The model under review builds one solid part; all positions refer to its coordinate system, in mm. A direction names the side the tool comes from. Round coordinates to 2 decimals unless told otherwise and drop trailing zeros. Loops run counter-clockwise (first coordinate to the right, second up) from the corner with the lowest first, then second, coordinate; pieces in that order, holes last. Notation, with made-up numbers: M 41.25,23 L 82.25,23 A26 cw 82.25,46 Z; hole C -10.5,61 d2. An arc over 180 degrees is marked long. Return JSON: item names as keys, results as strings. Group by question number.
Q1. Consider section B-B (y = -533.5). State the section outline as (x, z) points, and give its area (3 significant figures).
Q2. Consider section D-D (z = 609.5). State the section outline as (x, y) points, and give its area (3 significant figures).
Q3. Consider section A-A (x = 43). State the section outline as (y, z) points, and give its area (3 significant figures).
Q4. For faces 5 (the face through (-76.2, -9, 347)), 6 (the face through (-1, 590.55, 347)), list the 3-axis set-ups (+Z, -Z, +X, -X, +Y, -Y) from which the entire face can be reached by the end or side of a thin tool; tool diameter is ignored.
Q5. To check wall thickness, follow line 1 along Z through (x, y) = (61.5, 0); line 2 along X through (y, z) = (128.5, 73.5); line 3 along Y through (x, z) = (-68.75, 406.4). State the ranges of each line that lie inside material, in increasing order.
Q6. Consider section C-C (z = 268). State the section outline as (x, y) points.
Q7. Draft analysis for pull direction Y (two halves, no side actions). For faces 1 (the face through (62, 3, 0)), 2 (the face through (-1, -590.55, 347)), 3 (the face through (-1, 609.6, 347)), 4 (the face through (57.15, -8, 426)), state which applies: pulls with the +Y half, pulls with the -Y half, needs draft (parallel to the pull), parting line crosses it, or undercut.
from build123d import *

# Parameters (mm, degrees)
F0_W     = 152.4
F0_H     = 1219.2
F0_W_2   = 114.3
F0_H_2   = 1181.1
F1_DEPTH = 704.85
F3_DEPTH = 25.4
F5_DEPTH = 25.4


# Not quite as in the source:
# - a feature names something its author has since deleted; it is built from what else it names


with BuildPart() as f1:
    # F0 (on Top) → F1 (new body)
    with BuildSketch(Plane.XY):
        Rectangle(F0_W, F0_H)
        Rectangle(F0_W_2, F0_H_2, mode=Mode.SUBTRACT)
    extrude(amount=F1_DEPTH)

    # F2 (on face) → F3 (cut)
    with BuildSketch(Plane.YZ.offset(76.2)):
        with BuildLine():
            ThreePointArc((30.226, 596.9), (-21.3730095681, 618.2730095681), (0, 566.674))
            ThreePointArc((0, 566.674), (21.3730095681, 575.5269904319), (30.226, 596.9))
        make_face()
        Polygon((-133.35, 101.6), (0, 101.6), (133.35, 101.6), (133.35, 419.1), (0, 419.1), (-133.35, 419.1), align=None)
    extrude(amount=-F3_DEPTH, mode=Mode.SUBTRACT)

    # F4 (on face) → F5 (cut)
    with BuildSketch(Plane(origin=(-76.2, 0, 0), x_dir=(0, -1, 0), z_dir=(-1, 0, 0))):
        with BuildLine():
            ThreePointArc((30.226, 406.4), (-21.3730095681, 427.7730095681), (0, 376.174))
            ThreePointArc((0, 376.174), (21.3730095681, 385.0269904319), (30.226, 406.4))
        make_face()
    extrude(amount=-F5_DEPTH, mode=Mode.SUBTRACT)


solid = f1.part
Values:
{
 "1": {"outline": "M -76.2,0 L -57.15,0 L -57.15,704.85 L -76.2,704.85 Z; M 57.15,0 L 76.2,0 L 76.2,704.85 L 57.15,704.85 Z", "area": "26,900 mm2"},
 "2": {"outline": "M -76.2,-609.6 L 76.2,-609.6 L 76.2,-27.47 L 57.15,-27.47 L 57.15,-590.55 L -57.15,-590.55 L -57.15,590.55 L 57.15,590.55 L 57.15,27.47 L 76.2,27.47 L 76.2,609.6 L -76.2,609.6 Z", "area": "49,800 mm2"},
 "3": {"outline": "M -609.6,0 L -590.55,0 L -590.55,704.85 L -609.6,704.85 Z; M 590.55,0 L 609.6,0 L 609.6,704.85 L 590.55,704.85 Z", "area": "26,900 mm2"},
 "4": {"face 5": "+Z, -Z, -X, +Y, -Y", "face 6": "+Z, -Z"},
 "5": {"line 1": "z = 0 to 101.6, 419.1 to 566.67, 627.13 to 704.85", "line 2": "x = -76.2 to -57.15, 57.15 to 76.2", "line 3": "y = -609.6 to -30.23, 30.23 to 609.6"},
 "6": {"outline": "M -76.2,-609.6 L 76.2,-609.6 L 76.2,-133.35 L 57.15,-133.35 L 57.15,-590.55 L -57.15,-590.55 L -57.15,590.55 L 57.15,590.55 L 57.15,133.35 L 76.2,133.35 L 76.2,609.6 L -76.2,609.6 Z"},
 "7": {"face 1": "needs draft", "face 2": "undercut", "face 3": "pulls with the +Y half", "face 4": "undercut"}
}
